Design review of the part built by this model. Coordinates are the model's own, in mm. A direction names the side the tool comes from. Coordinates: 2 decimals unless noted, no trailing zeros. Write each loop counter-clockwise with the first axis right and the second up, starting at its lowest first coordinate (ties: lowest second). Pieces come first, ordered by that corner, then holes.
Q1. The part is to be moulded in two halves that separate along X. For faces 1 (the cylindrical face through (64.1, 8.8, 1)), 2 (the cylindrical face through (82.1, 51.14, -1.01)), 3 (the flat face through (41, 0, -1)), say which applies: released by +X, released by -X, zero draft, split by the parting line, or undercut.
Q2. For pin 1 Ø0.6 at (x, z) = (36, 1) entering from +Y; pin 2 Ø1.5 at (y, z) = (27, 1) entering from +X; pin 3 Ø5 at (x, y) = (37.5, 46.5) entering from +Z; pin 4 Ø1.9 at (x, y) = (78.5, 47.5) entering from -Z, all flat-tipped, find the tip position at first contact; note any pin that passes through.
Q3. For L1, parallel to Y at x = 64, z = 1.3 (1 decimal); L2, parallel to Y at x = 35, z = 0.8; L3, parallel to Y at x = 4.5, z = 0.65, list the stretches that pass through material, from the lowest coordinate up.
Q4. Take a section at A-A, the plane x = 78.5. Write out the cut boundary in (y, z), plus the area to 3 significant figures.
Q5. Take a section at C-C, the plane x = 26.5. Write out the cut boundary in (y, z).
Q6. Take a section at B-B, the plane x = 14. Write out the cut boundary in (y, z) (1 decimal).
Q7. For faces 4 (the flat face through (77, 25.05, 1)), 5 (the flat face through (41, 50, 1)), 6 (the cylindrical face through (81.43, 2.6, 1.01)), list the 3-axis set-ups (+Z, -Z, +X, -X, +Y, -Y) from which the entire face can be reached by the end or side of a thin tool; tool diameter is ignored.
from build123d import *

# Parameters (mm, degrees)
SKETCH_W             = 83
SKETCH_H             = 52
PAD_DEPTH            = 2
SKETCH001_W          = 30
SKETCH001_H          = 2
PAD001_DEPTH         = 2
SKETCH005_R          = 1.6
POCKET_DEPTH         = 5
POCKET_DEPTH_BACK    = -5
SKETCH003_R          = 1.375
POCKET001_DEPTH      = 2
POCKET001_DEPTH_BACK = 1.5
SKETCH004_W          = 1
SKETCH004_H          = 13
PAD002_DEPTH         = 2.5
CHAMFER_SIZE         = 1.95
FILLET_R             = 3
FILLET001_R          = 2


with BuildPart() as part:
    # Sketch → Pad (new body)
    with BuildSketch(Plane.XY):
        with Locations((41.5, 26)):
            Rectangle(SKETCH_W, SKETCH_H)
    extrude(amount=-PAD_DEPTH)

    # Sketch001 → Pad001 (join)
    with BuildSketch(Plane.XY):
        Polygon((2, 2), (2, 50), (82, 50), (82, 25.5), (83, 25.5), (83, 12), (82, 12), (82, 2), align=None)
        with BuildLine():
            Line((6.95, 47.997494), (76.05, 47.997494))
            ThreePointArc((76.05, 47.997494), (77.163963, 45.386944), (80, 45.5))
            Line((80, 25.05), (80, 45.5))
            Line((80, 25.05), (74.2, 25.05))
            Line((74.2, 25.05), (74.2, 11.55))
            Line((74.2, 11.55), (80, 11.55))
            Line((80, 11.55), (80, 6.5))
            ThreePointArc((80, 6.5), (77.163963, 6.613056), (76.05, 4.002506))
            Line((76.05, 4.002506), (66.401878, 4.002506))
            ThreePointArc((66.401878, 4.002506), (63.996871, 8.799998), (61.601878, 3.997499))
            Line((61.601878, 3.997499), (16.401878, 4.002506))
            ThreePointArc((16.401878, 4.002506), (13.996871, 8.799998), (11.601878, 3.997499))
            Line((11.601878, 3.997499), (6.951878, 3.9995))
            ThreePointArc((6.951878, 3.9995), (6.270443, 6.267581), (4.002506, 6.949493))
            Line((4.002506, 45.05), (4.002506, 6.949493))
            ThreePointArc((4.002506, 45.05), (6.267767, 45.732233), (6.95, 47.997494))
        make_face(mode=Mode.SUBTRACT)
        with Locations((40, 42)):
            Rectangle(SKETCH001_W, SKETCH001_H)
    extrude(amount=PAD001_DEPTH)

    # Sketch005 → Pocket (cut, two sides)
    with BuildSketch(Plane.XY) as pocket_sk:
        with Locations((4.5, 47.5)):
            Circle(SKETCH005_R)
        with Locations((78.5, 47.5)):
            Circle(SKETCH005_R)
        with Locations((78.5, 4.5)):
            Circle(SKETCH005_R)
        with Locations((4.5, 4.5)):
            Circle(SKETCH005_R)
    extrude(amount=-POCKET_DEPTH, mode=Mode.SUBTRACT)
    extrude(pocket_sk.sketch, amount=-POCKET_DEPTH_BACK, mode=Mode.SUBTRACT)

    # Sketch003 → Pocket001 (cut, two sides)
    with BuildSketch(Plane.XY.offset(0.5)) as pocket001_sk:
        with Locations((14, 5.8)):
            Circle(SKETCH003_R)
        with Locations((64, 5.8)):
            Circle(SKETCH003_R)
    extrude(amount=POCKET001_DEPTH, mode=Mode.SUBTRACT)
    extrude(pocket001_sk.sketch, amount=-POCKET001_DEPTH_BACK, mode=Mode.SUBTRACT)

    # Sketch004 → Pad002 (join)
    with BuildSketch(Plane.XY):
        with Locations((82.5, 19)):
            Rectangle(SKETCH004_W, SKETCH004_H)
    extrude(amount=PAD002_DEPTH)

    # Chamfer
    chamfer_edges = [part.edges().sort_by_distance(p)[0] for p in [
        (2.9, 47.5, -2),
        (2.9, 4.5, -2),
        (76.9, 4.5, -2),
        (76.9, 47.5, -2),
    ]]
    chamfer(chamfer_edges, length=CHAMFER_SIZE)

    # Fillet
    fillet_edges = [part.edges().sort_by_distance(p)[0] for p in [
        (83, 52, -1),
        (0, 52, -1),
        (0, 0, -1),
        (83, 0, -1),
    ]]
    fillet(fillet_edges, radius=FILLET_R)

    # Fillet001
    fillet001_edges = [part.edges().sort_by_distance(p)[0] for p in [
        (82, 2, 1),
        (2, 2, 1),
        (82, 50, 1),
        (2, 50, 1),
    ]]
    fillet(fillet001_edges, radius=FILLET001_R)


solid = part.part
Responses:
1. face 1: undercut
1. face 2: released by +X
1. face 3: zero draft
2. pin 1: stops at y = 50
2. pin 2: stops at x = 82
2. pin 3: stops at z = 2
2. pin 4: passes through
3. L1: y = 2 to 4.4, 7.2 to 8.8, 48 to 50
3. L2: y = 2 to 4, 41 to 43, 48 to 50
3. L3: y = 2 to 2.9, 6.1 to 7, 45 to 45.9, 49.1 to 50
4. outline: (0, -2) - (0.95, -2) - (2.9, -0.05) - (2.9, 2) - (2, 2) - (2, 0) - (0, 0) - close; (6.1, -0.05) - (8.05, -2) - (43.95, -2) - (45.9, -0.05) - (45.9, 2) - (45, 2) - (45, 0) - (25.05, 0) - (25.05, 2) - (11.55, 2) - (11.55, 0) - (7, 0) - (7, 2) - (6.1, 2) - close; (49.1, -0.05) - (51.05, -2) - (52, -2) - (52, 0) - (50, 0) - (50, 2) - (49.1, 2) - close
4. area: 118 mm2
5. outline: (0, -2) - (52, -2) - (52, 0) - (50, 0) - (50, 2) - (48, 2) - (48, 0) - (43, 0) - (43, 2) - (41, 2) - (41, 0) - (4, 0) - (4, 2) - (2, 2) - (2, 0) - (0, 0) - close
6. outline: (0, -2) - (52, -2) - (52, 0) - (50, 0) - (50, 2) - (48, 2) - (48, 0) - (8.8, 0) - (8.8, 2) - (7.2, 2) - (7.2, -1) - (4.4, -1) - (4.4, 2) - (2, 2) - (2, 0) - (0, 0) - close
7. face 4: +Z
7. face 5: +Z, +X, -X, +Y
7. face 6: +Z, +X, -Y
